Here's how the part is built. I have some questions about the finished solid (model axes, mm). Face numbers are marked on the shaded views. A direction names the side the tool comes from. Coordinates: 2 decimals unless noted, no trailing zeros. Write each loop counter-clockwise with the first axis right and the second up, starting at its lowest first coordinate (ties: lowest second). Pieces come first, ordered by that corner, then holes. Notation, with made-up numbers: (-33.5, -23.75) -> (0.5, -23.75) arc R20 cw to (0.5, -0.75) -> close; hole circle Ø4 at (57.5, -18). An arc over 180 degrees is marked (long way). Put each result on its own line as item: value.
```python
from build123d import *

# Parameters (mm, degrees)
F1_DEPTH = 1.27
F3_DEPTH = 12.7
F6_DEPTH = 1.778


with BuildPart() as f1:
    # F0 (on Top) → F1 (new body, symmetric)
    with BuildSketch(Plane.XY):
        with BuildLine():
            Line((0, 1.524), (0, 0))
            Line((0, 0), (12.7, 0))
            Line((12.7, 0), (12.7, -2.54))
            Line((12.7, -2.54), (4.572, -2.54))
            Line((4.572, -2.54), (4.572, -4.572))
            Line((4.572, -4.572), (12.5717104354, -4.572))
            ThreePointArc((12.5717104354, -4.572), (15.7940682602, -1.0438103752), (11.7644204026, 1.524))
            Line((11.7644204026, 1.524), (0, 1.524))
        make_face()
    extrude(amount=F1_DEPTH, both=True)

    # F2 (on face) → F3 (join, through all)
    with BuildSketch(Plane(origin=(0, 0, 0), x_dir=(0, -1, 0), z_dir=(-1, 0, 0))):
        Polygon((0.762, 0), (0, 0.508), (0, -0.508), align=None)
    extrude(amount=-F3_DEPTH)

    # F5 (on face) → F6 (join)
    with BuildSketch(Plane(origin=(0, 0, 0), x_dir=(0, -1, 0), z_dir=(-1, 0, 0))):
        Polygon((-4.064, -1.27), (-1.524, -1.27), (-1.524, 1.27), align=None)
    extrude(amount=-F6_DEPTH)


with BuildPart() as f7_1:
    # F7: copy of F1
    add(f1.part)


solid = f1.part
```
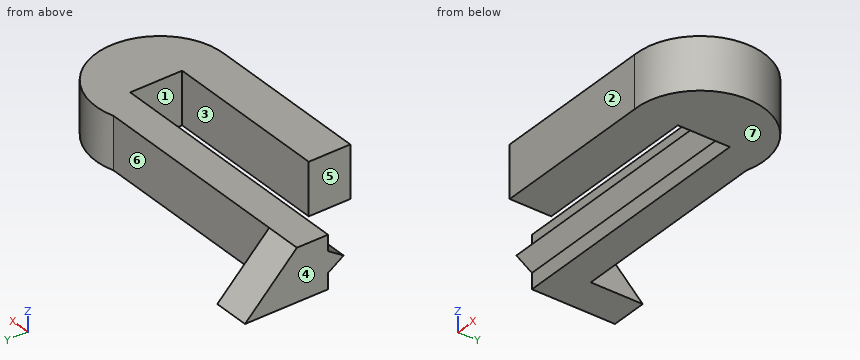
Item 1: Imagine slicing it at C-C on x = 4.25. Write out the boundary of the cut face in (y, z), then the cut area to 3 significant figures.
Output:
outline: (-0.76, 0) -> (0, -0.51) -> (0, -1.27) -> (1.52, -1.27) -> (1.52, 1.27) -> (0, 1.27) -> (0, 0.51) -> close
area: 4.26 mm²
Item 2: Imagine slicing it at A-A on x = 11. Write out the boundary of the cut face in (y, z).
Output:
outline: (-4.57, -1.27) -> (-2.54, -1.27) -> (-2.54, 1.27) -> (-4.57, 1.27) -> close; (-0.76, 0) -> (0, -0.51) -> (0, -1.27) -> (1.52, -1.27) -> (1.52, 1.27) -> (0, 1.27) -> (0, 0.51) -> close
Item 3: If we mould it in two halves opening along Y, with no side actions, what happens to the marked faces 1, 2, 3 and 4? For each: released by +Y, released by -Y, zero draft, split by the parting line, or undercut.
Output:
face 1: undercut
face 2: released by -Y
face 3: undercut
face 4: zero draft
Item 4: For P1, Ø0.8, axis at x = 4.5, z = -1, coming from the -Y side; P2, Ø1.5, axis at x = 3.5, z = 1, coming from the -Y side, each with a flat end and sliding along its axis, tell me the tip position at first contact or that it passes through.
Output:
P1: stops at y = -4.57
P2: stops at y = -0.39
Item 5: Imagine slicing it at D-D on y = 0.5. Write out the boundary of the cut face in (x, z), then the cut area to 3 significant figures.
Output:
outline: (0, -1.27) -> (15.13, -1.27) -> (15.13, 1.27) -> (0, 1.27) -> close
area: 38.4 mm²
Item 6: Please list where these lines run through material, in increasing order: line 1 along Y through (x, z) = (7.75, -0.7); line 2 along X through (y, z) = (3, -0.25); line 3 along Y through (x, z) = (5.75, -0.2). Write a range as from..to.
Output:
line 1: y = -4.57..-2.54, 0..1.52
line 2: x = 0..1.78
line 3: y = -4.57..-2.54, -0.46..1.52
Item 7: Which directions (+Z, -Z, +X, -X, +Y, -Y) give clear straight access to the entire face, cutting with the end or side of a thin tool? Please do the marked faces 5, 6 and 7.
Output:
face 5: +Z, -Z, -X, -Y
face 6: +Z, -Z, +Y
face 7: -Z, +X, -X, +Y, -Y
Item 8: Imagine slicing it at B-B on z = -0.95. Write out the boundary of the cut face in (x, y), then the cut area to 3 significant figures.
Output:
outline: (0, 0) -> (12.7, 0) -> (12.7, -2.54) -> (4.57, -2.54) -> (4.57, -4.57) -> (12.57, -4.57) arc R3.12 ccw (long way) to (11.76, 1.52) -> (1.78, 1.52) -> (1.78, 3.74) -> (0, 3.74) -> close
area: 55.2 mm²
